Build history of the part. All positions in model axes, mm. A direction names the side the tool comes from. Round coordinates to 2 decimals unless told otherwise and drop trailing zeros. Loops run counter-clockwise (first coordinate to the right, second up) from the corner with the lowest first, then second, coordinate; pieces in that order, holes last. Notation, with made-up numbers: (41.25, -5.75) -> (87.25, -5.75) arc R17 cw to (87.25, 4.25) -> close; hole circle Ø8 at (60.5, 11). An arc over 180 degrees is marked (long way). Put each result on its own line as item: value. Start each with the question number.
Item 1: Cut at C-C, the plane x = -27.5. List the corners of the cut face in (y, z).
Item 2: Cut at B-B, the plane z = 533.4. List the corners of the cut face in (x, y).
Item 3: Tool access for faces 4 (the flat face through (46.038, 1, 304)), 5 (the flat face through (50.8, -1, 304)): list every direction of +Z, -Z, +X, -X, +Y, -Y with a clear straight run to the whole face (end or side of a thin tool).
Item 4: Cut at A-A, the plane y = 0. List the corners of the cut face in (x, z).
Item 5: Drill centre lines: probe 1 along Z at (x, y) = (47, 0); probe 2 along Y at (x, z) = (-36, 67). Where is each one in solid material? Low to high. Write a range as [from, to].
Item 6: Pull direction Y, two halves, no side cores. Call faces 1 (the cylindrical face through (48.45, -1.72, 525.65)), 2 (the flat face through (-1, -50.8, 304)), 3 (the flat face through (-49, 0, 0)): +Y half, -Y half, draft (parallel to the pull), parting line (faces both ways), or undercut.
```python
from build123d import *

# Parameters (mm, degrees)
F1_DEPTH = 615.95
F3_DEPTH = 25.4
F4_R     = 7.9375
F5_DEPTH = 101.601


with BuildPart() as f1:
    # F0 (on Top) → F1 (new body)
    with BuildSketch(Plane.XY):
        with BuildLine():
            Line((43.65625, 50.8), (-43.65625, 50.8))
            ThreePointArc((-43.65625, 50.8), (-48.707644, 48.707644), (-50.8, 43.65625))
            Line((-50.8, 43.65625), (-50.8, -43.65625))
            ThreePointArc((-50.8, -43.65625), (-48.707644, -48.707644), (-43.65625, -50.8))
            Line((-43.65625, -50.8), (43.65625, -50.8))
            ThreePointArc((43.65625, -50.8), (48.707644, -48.707644), (50.8, -43.65625))
            Line((50.8, -43.65625), (50.8, 43.65625))
            ThreePointArc((50.8, 43.65625), (48.707644, 48.707644), (43.65625, 50.8))
        make_face()
        with BuildLine():
            Line((43.65625, -46.0375), (-43.65625, -46.0375))
            ThreePointArc((-43.65625, -46.0375), (-45.340048, -45.340048), (-46.0375, -43.65625))
            Line((-46.0375, -43.65625), (-46.0375, 43.65625))
            ThreePointArc((-46.0375, 43.65625), (-45.340048, 45.340048), (-43.65625, 46.0375))
            Line((-43.65625, 46.0375), (43.65625, 46.0375))
            ThreePointArc((43.65625, 46.0375), (45.340048, 45.340048), (46.0375, 43.65625))
            Line((46.0375, 43.65625), (46.0375, -43.65625))
            ThreePointArc((46.0375, -43.65625), (45.340048, -45.340048), (43.65625, -46.0375))
        make_face(mode=Mode.SUBTRACT)
    extrude(amount=F1_DEPTH)

    # F2 (on face) → F3 (cut)
    with BuildSketch(Plane.XZ.offset(50.8)):
        Polygon((-2.822954, 45.9105), (2.822954, 45.9105), (5.645908, 50.8), (2.822954, 55.6895), (-2.822954, 55.6895), (-5.645908, 50.8), align=None)
        Polygon((-2.822954, 204.6605), (2.822954, 204.6605), (5.645908, 209.55), (2.822954, 214.4395), (-2.822954, 214.4395), (-5.645908, 209.55), align=None)
        Polygon((-2.822954, 458.6605), (2.822954, 458.6605), (5.645908, 463.55), (2.822954, 468.4395), (-2.822954, 468.4395), (-5.645908, 463.55), align=None)
    extrude(amount=-F3_DEPTH, mode=Mode.SUBTRACT)

    # F4 (on face) → F5 (cut, through all)
    with BuildSketch(Plane.YZ.offset(50.8)):
        with Locations((0, 76.2)):
            Circle(F4_R)
        with Locations((0, 533.4)):
            Circle(F4_R)
    extrude(amount=-F5_DEPTH, mode=Mode.SUBTRACT)


solid = f1.part
```
Reply:
1. outline: (-50.8, 0) -> (-46.04, 0) -> (-46.04, 615.95) -> (-50.8, 615.95) -> close; (46.04, 0) -> (50.8, 0) -> (50.8, 615.95) -> (46.04, 615.95) -> close
2. outline: (-50.8, -43.66) arc R7.14 ccw to (-43.66, -50.8) -> (43.66, -50.8) arc R7.14 ccw to (50.8, -43.66) -> (50.8, -7.94) -> (46.04, -7.94) -> (46.04, -43.66) arc R2.38 cw to (43.66, -46.04) -> (-43.66, -46.04) arc R2.38 cw to (-46.04, -43.66) -> (-46.04, -7.94) -> (-50.8, -7.94) -> close; (-50.8, 7.94) -> (-46.04, 7.94) -> (-46.04, 43.66) arc R2.38 cw to (-43.66, 46.04) -> (43.66, 46.04) arc R2.38 cw to (46.04, 43.66) -> (46.04, 7.94) -> (50.8, 7.94) -> (50.8, 43.66) arc R7.14 ccw to (43.66, 50.8) -> (-43.66, 50.8) arc R7.14 ccw to (-50.8, 43.66) -> close
3. face 4: +Z, -Z
3. face 5: +Z, -Z, +X, +Y, -Y
4. outline: (-50.8, 0) -> (-46.04, 0) -> (-46.04, 68.26) -> (-50.8, 68.26) -> close; (-50.8, 84.14) -> (-46.04, 84.14) -> (-46.04, 525.46) -> (-50.8, 525.46) -> close; (-50.8, 541.34) -> (-46.04, 541.34) -> (-46.04, 615.95) -> (-50.8, 615.95) -> close; (46.04, 0) -> (50.8, 0) -> (50.8, 68.26) -> (46.04, 68.26) -> close; (46.04, 84.14) -> (50.8, 84.14) -> (50.8, 525.46) -> (46.04, 525.46) -> close; (46.04, 541.34) -> (50.8, 541.34) -> (50.8, 615.95) -> (46.04, 615.95) -> close
5. probe 1: z = [0, 68.26], [84.14, 525.46], [541.34, 615.95]
5. probe 2: y = [-50.8, -46.04], [46.04, 50.8]
6. face 1: undercut
6. face 2: -Y half
6. face 3: draft
